The model under review builds one solid part; all positions refer to its coordinate system, in mm. A direction names the side the tool comes from. Coordinates: 2 decimals unless noted, no trailing zeros. Write each loop counter-clockwise with the first axis right and the second up, starting at its lowest first coordinate (ties: lowest second). Pieces come first, ordered by that corner, then holes.
1) For line 1 (Z direction, x = 3.5, y = 15); line 2 (Y direction, x = 12, z = -19.25); line 3 (Y direction, x = 4, z = -5.25), list the stretches that pass through material, from the lowest coordinate up.
2) Machinability: for faces 4 (the flat face through (14, 11, -19.6)), 5 (the flat face through (19, 8, 0)), which of the approach directions +Z, -Z, +X, -X, +Y, -Y give a long, thin tool a straight path to every point of the face, cutting with its end or side? Answer none if there is none.
3) Add section C-C, the plane z = -12.25. State the section outline as (x, y) points.
4) Mouldability with a two-part tool opening along Z and no side actions: class faces 1 (the cylindrical face through (20.385, 4.882, -10.726)), 2 (the flat face through (19, -1.6, -10)), 3 (the flat face through (19, 8, -21.2)) as released by +Z, released by -Z, zero draft, split by the parting line, or undercut.
5) Add section A-A, the plane x = 10.5. State the section outline as (y, z) points, then the cut area to 3 significant figures.
6) Add section B-B, the plane y = 5.75. State the section outline as (x, z) points.
Autodesk Inventor part; units mm, degrees
ref_plane "YZ Plane" through (0, 0, 0) normal (1, 0, 0) x (0, 1, 0)
ref_plane "XZ Plane" through (0, 0, 0) normal (0, 1, 0) x (-1, 0, 0)
ref_plane "XY Plane" through (0, 0, 0) normal (0, 0, 1) x (1, 0, 0)
sketch "Esboço1" plane through (0, 0, 0) normal (0, 1, 0) x (-1, 0, 0)
  line L0 (-36, -1.6) -> (0, -1.6)
  line L1 (0, -19.6) -> (-36, -19.6)
  line L2 (-36, -19.6) -> (-36, -1.6)
  line L3 (0, 0) -> (-37.6, 0)
  line L4 (-37.6, 0) -> (-37.6, -21.2)
  line L5 (-37.6, -21.2) -> (0, -21.2)
  line L6 (0, -21.2) -> (0, 0)
  dimension "d0" = 1.6
  dimension "d1" = 18
  dimension "d7" = 36
sketch "Esboço1 outline for Extrusão1" plane through (0, 0, 0) normal (0, 1, 0) x (-1, 0, 0)
  line L0 (0, -21.2) -> (0, 0)
  line L1 (-37.6, -21.2) -> (0, -21.2)
  line L2 (-37.6, 0) -> (-37.6, -21.2)
  line L3 (0, 0) -> (-37.6, 0)
extrude "Extrusão1" add sketch "Esboço1 outline for Extrusão1" against normal blind 1.6
sketch "Esboço1 outline for Extrusão2" plane through (0, 0, 0) normal (0, 1, 0) x (-1, 0, 0)
  line L0 (-36, -19.6) -> (-36, -1.6)
  line L1 (0, -19.6) -> (-36, -19.6)
  line L2 (0, -21.2) -> (0, -19.6)
  line L3 (-37.6, -21.2) -> (0, -21.2)
  line L4 (-37.6, 0) -> (-37.6, -21.2)
  line L5 (0, 0) -> (-37.6, 0)
  line L6 (0, -1.6) -> (0, 0)
  line L7 (-36, -1.6) -> (0, -1.6)
extrude "Extrusão2" add sketch "Esboço1 outline for Extrusão2" along normal blind 18
fillet "Arredondamento1" radius 45 1 edges at (36, 0, -10.6)
equation "\"d0\" = Margem"
equation "\"d1\" = Esfera"
equation "\"d7\" = 2 * Esfera"
equation "\"d2\" = Margem"
equation "\"d4\" = Esfera"
equation "\"d6\" = 2.5 * Esfera"
equation "\"Esfera\" = 18"
equation "\"Margem\" = 1.6"
properties part number "Peça que libera"
Geometry results:
1. line 1: z = -21.2 to -19.6, -1.6 to 0
1. line 2: y = -1.6 to 1.63
1. line 3: y = -1.6 to 0.18
2. face 4: -X, +Y
2. face 5: +Z, +X, -X, +Y, -Y
3. outline: (0, -1.6) - (37.6, -1.6) - (37.6, 18) - (36, 18) arc R45 cw to (0, 0) - close
4. face 1: undercut
4. face 2: zero draft
4. face 3: released by -Z
5. outline: (-1.6, -21.2) - (18, -21.2) - (18, -19.6) - (1.24, -19.6) - (1.24, -1.6) - (18, -1.6) - (18, 0) - (-1.6, 0) - close
5. area: 114 mm2
6. outline: (0, -21.2) - (37.6, -21.2) - (37.6, 0) - (0, 0) - (0, -1.6) - (22.01, -1.6) - (22.01, -19.6) - (0, -19.6) - close
